Study the drawing (mm; zero at the part's minimum x, y, z) and answer. Coordinates: 2 decimals unless noted, no trailing zeros. Order: outer loops, then holes, each group sorted by start corner. A loop starts at its lowest first (then second) coordinate and runs counter-clockwise, first axis right, second up.
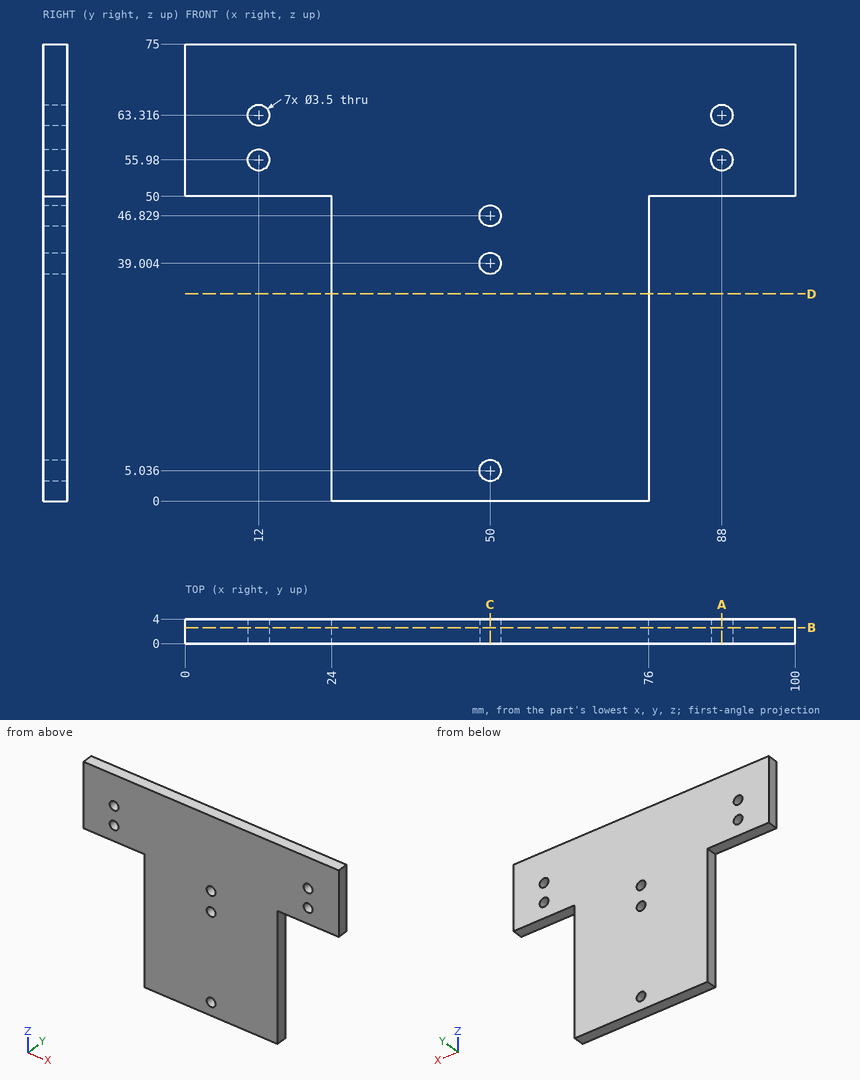
1) A cutting plane is placed at A-A, the plane x = 88. Determine the outline of the cut face in (y, z), and give its area (3 significant figures).
A:
outline: (0, 50) - (4, 50) - (4, 54.23) - (0, 54.23) - close; (0, 57.73) - (4, 57.73) - (4, 61.57) - (0, 61.57) - close; (0, 65.07) - (4, 65.07) - (4, 75) - (0, 75) - close
area: 72.0 mm2
2) A cutting plane is placed at C-C, the plane x = 50. Determine the outline of the cut face in (y, z).
A:
outline: (0, 0) - (4, 0) - (4, 3.29) - (0, 3.29) - close; (0, 6.79) - (4, 6.79) - (4, 37.25) - (0, 37.25) - close; (0, 40.75) - (4, 40.75) - (4, 45.08) - (0, 45.08) - close; (0, 48.58) - (4, 48.58) - (4, 75) - (0, 75) - close
3) Flat-ended cylindrical pins translate along their axes: pin 1 Ø1.2 at (y, z) = (2, 14.5) entering from -X; pin 2 Ø2 at (x, z) = (50, 46.83) entering from +Y; pin 3 Ø2 at (x, y) = (6.5, 2) entering from -Z; pin 4 Ø2 at (y, z) = (2, 8.5) entering from +X. Find the tip coordinate at first contact, or state that the pin passes through.
A:
pin 1: stops at x = 24
pin 2: passes through
pin 3: stops at z = 50
pin 4: stops at x = 76
4) A cutting plane is placed at B-B, the plane y = 2.6. Determine the outline of the cut face in (x, z), and give its area (3 significant figures).
A:
outline: (0, 50) - (24, 50) - (24, 0) - (76, 0) - (76, 50) - (100, 50) - (100, 75) - (0, 75) - close; hole circle Ø3.5 at (12, 55.98); hole circle Ø3.5 at (12, 63.32); hole circle Ø3.5 at (50, 5.04); hole circle Ø3.5 at (50, 39); hole circle Ø3.5 at (50, 46.83); hole circle Ø3.5 at (88, 55.98); hole circle Ø3.5 at (88, 63.32)
area: 5,030 mm2
5) Straight lines are drawn through the part: line 1 (Z direction, x = 88, y = 2.05); line 2 (X direction, y = 2.45, z = 63.5); line 3 (Z direction, x = 11.5, y = 2.35). For each, find the intervals that lie inside material, in ascending order.
A:
line 1: z = 50 to 54.23, 57.73 to 61.57, 65.07 to 75
line 2: x = 0 to 10.26, 13.74 to 86.26, 89.74 to 100
line 3: z = 50 to 54.3, 57.66 to 61.64, 64.99 to 75
6) A cutting plane is placed at D-D, the plane z = 34. Determine the outline of the cut face in (x, y).
A:
outline: (24, 0) - (76, 0) - (76, 4) - (24, 4) - close
